Autodesk Inventor part; units mm, degrees
ref_plane "YZ Plane" through (0, 0, 0) normal (1, 0, 0) x (0, 1, 0)
ref_plane "XZ Plane" through (0, 0, 0) normal (0, 1, 0) x (-1, 0, 0)
ref_plane "XY Plane" through (0, 0, 0) normal (0, 0, 1) x (1, 0, 0)
sketch "Sketch1" plane through (0, 0, 0) normal (1, 0, 0) x (0, 1, 0)
  circle A0 centre (0, 0) radius 3.175
  dimension "d0" = 6.35
extrude "Extrusion1" add sketch "Sketch1" along normal blind 19.3548
ref_plane "Work Plane1" through (1.143, 0, 0) normal (-1, 0, 0) x (0, 0, 1)
sketch "Sketch2" plane through (1.143, 0, 0) normal (-1, 0, 0) x (0, 0, 1)
  circle A0 centre (0, 0) radius 3.175
  circle A1 centre (0, 0) radius 2.9845
  dimension "d4" = 5.969
extrude "Extrusion2" cut sketch "Sketch2" against normal blind 0.762
sketch "Sketch3" plane through (19.3548, 0, 0) normal (1, 0, 0) x (0, 0, -1)
  circle A0 centre (0, 0) radius 3.175
hole "Hole1" at (19.3548, 0, 0) direction (-1, 0, 0) diameter 5.08 depth 14.351
sketch "Sketch4" plane through (0, 0, 0) normal (-1, 0, 0) x (0, 0, 1)
  circle A0 centre (0, 0) radius 3.175
  line L0 (0, 1.2065) -> (1.0449, 0.6033)
  line L1 (1.0449, 0.6033) -> (1.0449, -0.6033)
  line L2 (1.0449, -0.6033) -> (0, -1.2065)
  line L3 (0, -1.2065) -> (-1.0449, -0.6033)
  line L4 (-1.0449, -0.6033) -> (-1.0449, 0.6032)
  line L5 (-1.0449, 0.6032) -> (0, 1.2065)
  dimension "d15" = 2.413
extrude "Extrusion3" cut sketch "Sketch4" against normal through all contours L0 L1 L2 L3 L4 L5
thread "Thread1"
properties part number "Clutch Sleeve2" material "Steel"
Can you work these out from the model? Positions are in its coordinate system, mm. A direction names the side the tool comes from. Round coordinates to 2 decimals unless told otherwise and drop trailing zeros. Order: outer loops, then holes, each group sorted by start corner. A loop starts at its lowest first (then second) coordinate and runs counter-clockwise, first axis right, second up.
(1) If we section it at C-C (x = 10.5): Please give me the cut outline in (y, z) (3 decimals), plus the area to 3 significant figures.
Results are:
outline: circle Ø6.35 at (0, 0); hole circle Ø5.08 at (0, 0)
area: 11.4 mm2
(2) If we section it at A-A (y = -0.25): Please give me the cut outline in (x, z) (3 decimals).
Results are:
outline: (0, -3.165) - (1.143, -3.165) - (1.143, -2.974) - (1.905, -2.974) - (1.905, -3.165) - (19.355, -3.165) - (19.355, -2.528) - (5.004, -2.528) - (5.004, -1.045) - (0, -1.045) - close; (0, 1.045) - (5.004, 1.045) - (5.004, 2.528) - (19.355, 2.528) - (19.355, 3.165) - (1.905, 3.165) - (1.905, 2.974) - (1.143, 2.974) - (1.143, 3.165) - (0, 3.165) - close
(3) If we section it at B-B (z = -0.75): Please give me the cut outline in (x, y) (3 decimals).
Results are:
outline: (0, -3.085) - (1.143, -3.085) - (1.143, -2.889) - (1.905, -2.889) - (1.905, -3.085) - (19.355, -3.085) - (19.355, -2.427) - (5.004, -2.427) - (5.004, -0.774) - (0, -0.774) - close; (0, 0.773) - (5.004, 0.773) - (5.004, 2.427) - (19.355, 2.427) - (19.355, 3.085) - (1.905, 3.085) - (1.905, 2.889) - (1.143, 2.889) - (1.143, 3.085) - (0, 3.085) - close
(4) If I drill on L1, parallel to Y at x = 10.75, z = 0 (3 decimals); L2, parallel to Z at x = 3.5, y = 0 (3 decimals), over which ranges is the centre line in solid material (lowest first)?
Results are:
L1: y = -3.175 to -2.54, 2.54 to 3.175
L2: z = -3.175 to -1.045, 1.045 to 3.175
(5) If we section it at D-D (y = 1.75): Please give me the cut outline in (x, z) (3 decimals), plus the area to 3 significant figures.
Results are:
outline: (0, -2.649) - (1.143, -2.649) - (1.143, -2.418) - (1.905, -2.418) - (1.905, -2.649) - (19.355, -2.649) - (19.355, -1.841) - (5.004, -1.841) - (5.004, 1.841) - (19.355, 1.841) - (19.355, 2.649) - (1.905, 2.649) - (1.905, 2.418) - (1.143, 2.418) - (1.143, 2.649) - (0, 2.649) - close
area: 49.4 mm2
(6) On a 3-axis mill with a long thin cutter (end or side, diameter ignored), from which of +Z, -Z, +X, -X, +Y, -Y can I reach the whole of each face in a straight line? I mean faces 4 (the face through (2.467, -0.909, -0.515)), 5 (the face through (1.519, -2.914, -0.647)), 6 (the face through (5.004, 1, -1)), 7 (the face through (0, 1.4, 0)). Say none if no direction works.
Results are:
face 4: +X, -X
face 5: none
face 6: +X
face 7: +Z, -Z, -X, +Y, -Y
(7) We'd pull the mould along Z, two halves only. Please class faces 1 (the face through (10.51, -0.69, 3.1)), 2 (the face through (19.355, 0, 3)), 3 (the face through (2.47, -0.9, 0.53)): +Z half, -Z half, draft (parallel to the pull), parting line (faces both ways), or undercut.
Results are:
face 1: parting line
face 2: draft
face 3: undercut
(8) I'm going to push flat-ended pins straight in: pin 1 (1 mm diameter, centred on x = 7, z = 2, fed in from +Y); pin 2 (2 mm diameter, centred on x = 8, z = 2, fed in from -Y); pin 3 (1.5 mm diameter, centred on y = 1, z = 0, fed in from +X). Where does each tip first touch, or does it pass through?
Results are:
pin 1: stops at y = 2.8
pin 2: stops at y = -3.01
pin 3: stops at x = 5
